Read the model definition and answer for the solid it produces. Units are mm, in the model's axes. A direction names the side the tool comes from. Coordinates: 2 decimals unless noted, no trailing zeros. Order: outer loops, then holes, each group sorted by start corner. A loop starts at its lowest first (then second) coordinate and runs counter-clockwise, first axis right, second up. Notation, with made-up numbers: M 43,53.25 L 54,53.25 A25 cw 54,69.25 Z; hole C 24.5,84.5 d5. An arc over 180 degrees is marked long. One line per question, with ' | ' between items. Start each with the question number.
1) Consider probe 1 along Z at (x, y) = (15.5, 0); probe 2 along Z at (x, y) = (18.75, 41.5); probe 3 along X at (y, z) = (6.5, -39.5). Determine where each line is inside the solid, lowest interval first.
2) A tool of negligible diameter and unlimited length cuts with its end or side. For faces 1 (the face through (3.219, -6.883, 30.995)), 2 (the face through (18.96, -43.19, -62.11)), 3 (the face through (19.139, -100.788, -12.819)), 4 (the face through (19, 75, -6.35)), 5 (the face through (19.139, -39.458, 93.625)), from which of +Z, -Z, +X, -X, +Y, -Y can it reach the whole face along a straight path? Write none if from no direction.
3) Find section A-A, the plane z = 0. Write down the section's boundary in (x, y).
4) Given P1, Ø12, axis at x = 5.5, y = -68.5, coming from the +Z side; P2, Ø2, axis at x = 12.5, y = 55.5, coming from the -Z side; P3, Ø4, axis at x = 9.5, y = 22.5, coming from the +Z side; P4, Ø5, axis at x = 11.5, y = 59.5, coming from the +Z side, each flat-ended and moving along its own axis, determine where each tip first touches the part or whether it passes through.
5) Find section B-B, the plane y = 0. Write down the section's boundary in (x, z), plus the area to 3 significant figures.
6) Find section D-D, the plane x = 9.75. Write down the section's boundary in (y, z), plus the area to 3 significant figures.
7) Find section C-C, the plane z = 43.5. Write down the section's boundary in (x, y), plus the area to 3 significant figures.
from build123d import *

# Parameters (mm, degrees)
SKETCH2_R          = 19.05
CUT_EXTRUDE1_DEPTH = 26.4
SKETCH3_R          = 38.1
CUT_EXTRUDE2_DEPTH = 13.7
CUT_EXTRUDE5_DEPTH = 13.7
SKETCH6_W          = 9.144
SKETCH6_H          = 5.08
CUT_EXTRUDE6_DEPTH = 26.4


with BuildPart() as part:
    # Sketch1 → Revolve1 (revolve)
    with BuildSketch(Plane.XY):
        with BuildLine():
            Line((0, 0), (0, 31.75))
            Line((0, 31.75), (6.35, 31.75))
            ThreePointArc((6.35, 31.75), (10.840128061, 33.609871939), (12.7, 38.1))
            Line((12.7, 38.1), (12.7, 101.6))
            Line((12.7, 101.6), (25.4, 101.6))
            Line((25.4, 101.6), (25.4, 0))
            Line((25.4, 0), (0, 0))
        make_face()
    revolve(axis=Axis((25.4, 0, 0), (-1, 0, 0)))

    # Sketch2 → Cut-Extrude1 (cut, through all)
    with BuildSketch(Plane.ZY):
        Circle(SKETCH2_R)
    extrude(amount=-CUT_EXTRUDE1_DEPTH, mode=Mode.SUBTRACT)

    # Sketch3 → Cut-Extrude2 (cut, through all)
    with BuildSketch(Plane.ZY.offset(-12.7)):
        with Locations((114.3, 0)):
            Circle(SKETCH3_R)
        with Locations((57.15, -98.986703653)):
            Circle(SKETCH3_R)
        with Locations((-57.15, -98.986703653)):
            Circle(SKETCH3_R)
        with Locations((-114.3, 0)):
            Circle(SKETCH3_R)
        with Locations((-57.15, 98.986703653)):
            Circle(SKETCH3_R)
        with Locations((57.15, 98.986703653)):
            Circle(SKETCH3_R)
    extrude(amount=-CUT_EXTRUDE2_DEPTH, mode=Mode.SUBTRACT)

    # Sketch5 → Cut-Extrude5 (cut, through all)
    with BuildSketch(Plane.ZY.offset(-12.7)):
        with BuildLine():
            Line((113.723029824, 58.325673463), (46.547661143, 19.541956272))
            ThreePointArc((46.547661143, 19.541956272), (37.873399829, 21.866217586), (40.197661143, 30.5404789))
            Line((40.197661143, 30.5404789), (107.373029824, 69.324196091))
            Line((107.373029824, 69.324196091), (113.723029824, 58.325673463))
        make_face()
        with BuildLine():
            Line((-6.35, 127.649869555), (6.35, 127.649869555))
            Line((6.35, 127.649869555), (6.35, 50.082435173))
            ThreePointArc((6.35, 50.082435173), (0, 43.732435173), (-6.35, 50.082435173))
            Line((-6.35, 50.082435173), (-6.35, 127.649869555))
        make_face()
        with BuildLine():
            Line((107.373029824, -69.324196091), (40.197661143, -30.5404789))
            ThreePointArc((40.197661143, -30.5404789), (37.873399829, -21.866217586), (46.547661143, -19.541956272))
            Line((46.547661143, -19.541956272), (113.723029824, -58.325673463))
            Line((113.723029824, -58.325673463), (107.373029824, -69.324196091))
        make_face()
        with BuildLine():
            Line((-6.35, -127.649869555), (-6.35, -50.082435173))
            ThreePointArc((-6.35, -50.082435173), (0, -43.732435173), (6.35, -50.082435173))
            Line((6.35, -50.082435173), (6.35, -127.649869555))
            Line((6.35, -127.649869555), (-6.35, -127.649869555))
        make_face()
        with BuildLine():
            Line((-113.723029824, -58.325673463), (-46.547661143, -19.541956272))
            ThreePointArc((-46.547661143, -19.541956272), (-37.873399829, -21.866217586), (-40.197661143, -30.5404789))
            Line((-40.197661143, -30.5404789), (-107.373029824, -69.324196091))
            Line((-107.373029824, -69.324196091), (-113.723029824, -58.325673463))
        make_face()
        with BuildLine():
            Line((-107.373029824, 69.324196091), (-40.197661143, 30.5404789))
            ThreePointArc((-40.197661143, 30.5404789), (-37.873399829, 21.866217586), (-46.547661143, 19.541956272))
            Line((-46.547661143, 19.541956272), (-113.723029824, 58.325673463))
            Line((-113.723029824, 58.325673463), (-107.373029824, 69.324196091))
        make_face()
    extrude(amount=-CUT_EXTRUDE5_DEPTH, mode=Mode.SUBTRACT)

    # Sketch6 → Cut-Extrude6 (cut, through all)
    with BuildSketch(Plane.ZY):
        with Locations((0, 21.033223516)):
            Rectangle(SKETCH6_W, SKETCH6_H)
    extrude(amount=-CUT_EXTRUDE6_DEPTH, mode=Mode.SUBTRACT)


solid = part.part
Report:
1) probe 1: z = -76.2 to -19.05, 19.05 to 76.2 | probe 2: z = -92.74 to -84.58, -59.18 to 59.18, 84.58 to 92.74 | probe 3: x = 12.7 to 25.4
2) face 1: -X | face 2: +X, -X | face 3: -Z, +X, -X, -Y | face 4: +X, -X, +Y | face 5: +Z, +X, -X, -Y
3) outline: M 0,-31.75 L 6.35,-31.75 A6.35 cw 12.7,-38.1 L 12.7,-43.73 L 25.4,-43.73 L 25.4,-19.05 L 0,-19.05 Z; M 0,23.57 L 25.4,23.57 L 25.4,43.73 L 12.7,43.73 L 12.7,38.1 A6.35 cw 6.35,31.75 L 0,31.75 Z
4) P1: passes through | P2: stops at z = -84.64 | P3: stops at z = 26.39 | P4: stops at z = 83.9
5) outline: M 0,-31.75 L 6.35,-31.75 A6.35 cw 12.7,-38.1 L 12.7,-76.2 L 25.4,-76.2 L 25.4,-19.05 L 0,-19.05 Z; M 0,19.05 L 25.4,19.05 L 25.4,76.2 L 12.7,76.2 L 12.7,38.1 A6.35 cw 6.35,31.75 L 0,31.75 Z | area: 1,790 mm^2
6) outline: C 0,0 d65.47; hole M 18.49,-4.57 L 23.57,-4.57 L 23.57,4.57 L 18.49,4.57 A19.05 ccw long Z | area: 2,180 mm^2
7) outline: M 12.7,-63.42 L 25.4,-63.42 L 25.4,-32.45 L 12.7,-32.45 Z; M 12.7,-18.69 L 25.4,-18.69 L 25.4,18.69 L 12.7,18.69 Z; M 12.7,32.45 L 25.4,32.45 L 25.4,63.42 L 12.7,63.42 Z | area: 1,260 mm^2
